from build123d import *

# Parameters (mm, degrees)
BOSS_EXTRUDE1_DEPTH             = 9
SKETCH2_R                       = 15
MOTOR_HOLE_DEPTH                = 123.513264588
CBORE_START                     = -1
CBORE_SLOT_FOR_M3_SHCS1_DEPTH   = 10
CBORE_START_2                   = 6
CBORE_SLOT_FOR_M3_SHCS1_2_DEPTH = 3
LPATTERN2_COUNT                 = 2
LPATTERN2_PITCH                 = 31
LPATTERN2_COUNT_DIR2            = 2
LPATTERN2_PITCH_DIR2            = 31
CBORE_SLOT_FOR_M5_SHCS1_DEPTH   = 5
CBORE_START_3                   = 5
CBORE_SLOT_FOR_M5_SHCS1_2_DEPTH = 4
M5X0_8_TAPPED_HOLE1_D           = 4.2


with BuildPart() as part:
    # Sketch1 → Boss-Extrude1 (new body)
    with BuildSketch(Plane.XY):
        Polygon((-33.5, 0), (33.5, 0), (33.5, 117.5), (-28.5, 117.5), (-33.5, 112.5), align=None)
    extrude(amount=BOSS_EXTRUDE1_DEPTH)

    # Sketch2 → Motor Hole (cut, through all)
    with BuildSketch(Plane.XY.offset(9)):
        with Locations((0, 44.5)):
            Circle(SKETCH2_R)
    extrude(amount=-MOTOR_HOLE_DEPTH, mode=Mode.SUBTRACT)

    # CBORE SLOT for M3 SHCS1: read off the stored shape, not the designer's step
    # CBORE SLOT for M3 SHCS1 outline → CBORE SLOT for M3 SHCS1 (cut)
    with BuildSketch(Plane.XY.offset(CBORE_START)):
        with BuildLine():
            Line((-13.8, 55.2), (-13.8, 65.3))
            ThreePointArc((-13.8, 65.3), (-15.5, 67), (-17.2, 65.3))
            Line((-17.2, 65.3), (-17.2, 55.2))
            ThreePointArc((-17.2, 55.2), (-15.5, 53.5), (-13.8, 55.2))
        make_face()
    cbore_slot_for_m3_shcs1 = extrude(amount=CBORE_SLOT_FOR_M3_SHCS1_DEPTH, mode=Mode.SUBTRACT)

    # CBORE SLOT for M3 SHCS1 2 outline → CBORE SLOT for M3 SHCS1 2 (cut)
    with BuildSketch(Plane.XY.offset(CBORE_START_2)):
        with BuildLine():
            Line((-12.25, 55.2), (-12.25, 65.3))
            ThreePointArc((-12.25, 65.3), (-15.5, 68.55), (-18.75, 65.3))
            Line((-18.75, 65.3), (-18.75, 55.2))
            ThreePointArc((-18.75, 55.2), (-15.5, 51.95), (-12.25, 55.2))
        make_face()
        with BuildLine():
            ThreePointArc((-17.2, 65.3), (-15.5, 67), (-13.8, 65.3))
            Line((-13.8, 65.3), (-13.8, 55.2))
            ThreePointArc((-13.8, 55.2), (-15.5, 53.5), (-17.2, 55.2))
            Line((-17.2, 55.2), (-17.2, 65.3))
        make_face(mode=Mode.SUBTRACT)
    cbore_slot_for_m3_shcs1_2 = extrude(amount=CBORE_SLOT_FOR_M3_SHCS1_2_DEPTH, mode=Mode.SUBTRACT)

    # CBORE SLOT for M3 SHCS1 3: loft between two sections, ruled curve by curve
    cbore_slot_for_m3_shcs1_3_from = [
        Edge.make_three_point_arc((-12.25, 65.3, 8.975), (-13.201902961, 67.598097039, 8.975), (-15.5, 68.55, 8.975)),
        Edge.make_three_point_arc((-15.5, 68.55, 8.975), (-17.798097039, 67.598097039, 8.975), (-18.75, 65.3, 8.975)),
        Edge.make_three_point_arc((-18.75, 55.2, 8.975), (-17.798097039, 52.901902961, 8.975), (-15.5, 51.95, 8.975)),
        Edge.make_three_point_arc((-15.5, 51.95, 8.975), (-13.201902961, 52.901902961, 8.975), (-12.25, 55.2, 8.975)),
        Edge.make_line((-18.75, 65.3, 8.975), (-18.75, 55.2, 8.975)),
        Edge.make_line((-12.25, 65.3, 8.975), (-12.25, 55.2, 8.975)),
    ]
    cbore_slot_for_m3_shcs1_3_to = [
        Edge.make_three_point_arc((-12.225, 65.3, 9), (-13.184225292, 67.615774708, 9), (-15.5, 68.575, 9)),
        Edge.make_three_point_arc((-15.5, 68.575, 9), (-17.815774708, 67.615774708, 9), (-18.775, 65.3, 9)),
        Edge.make_three_point_arc((-18.775, 55.2, 9), (-17.815774708, 52.884225292, 9), (-15.5, 51.925, 9)),
        Edge.make_three_point_arc((-15.5, 51.925, 9), (-13.184225292, 52.884225292, 9), (-12.225, 55.2, 9)),
        Edge.make_line((-18.775, 65.3, 9), (-18.775, 55.2, 9)),
        Edge.make_line((-12.225, 65.3, 9), (-12.225, 55.2, 9)),
    ]
    cbore_slot_for_m3_shcs1_3 = Solid(Shell([*[Face.make_surface_from_curves(cbore_slot_for_m3_shcs1_3_from[k], cbore_slot_for_m3_shcs1_3_to[k]) for k in range(6)], Face(Wire(cbore_slot_for_m3_shcs1_3_from)), Face(Wire(cbore_slot_for_m3_shcs1_3_to))]))
    add(cbore_slot_for_m3_shcs1_3, mode=Mode.SUBTRACT)

    # LPattern2: CBORE SLOT for M3 SHCS1, CBORE SLOT for M3 SHCS1 2, CBORE SLOT for M3 SHCS1 3 2 × 2
    with Locations(*[(i * LPATTERN2_PITCH, -j * LPATTERN2_PITCH_DIR2, 0) for i in range(LPATTERN2_COUNT) for j in range(LPATTERN2_COUNT_DIR2) if (i, j) != (0, 0)]):
        add(cbore_slot_for_m3_shcs1, mode=Mode.SUBTRACT)
        add(cbore_slot_for_m3_shcs1_2, mode=Mode.SUBTRACT)
        add(cbore_slot_for_m3_shcs1_3, mode=Mode.SUBTRACT)

    # CBORE SLOT for M5 SHCS1: read off the stored shape, not the designer's step
    # CBORE SLOT for M5 SHCS1 outline → CBORE SLOT for M5 SHCS1 (cut)
    with BuildSketch(Plane.XY):
        with BuildLine():
            ThreePointArc((20.5, 42.5), (25.5, 37.5), (30.5, 42.5))
            Line((30.5, 42.5), (30.5, 57.5))
            ThreePointArc((30.5, 57.5), (25.5, 62.5), (20.5, 57.5))
            Line((20.5, 57.5), (20.5, 42.5))
        make_face()
    cbore_slot_for_m5_shcs1 = extrude(amount=CBORE_SLOT_FOR_M5_SHCS1_DEPTH, mode=Mode.SUBTRACT)

    # CBORE SLOT for M5 SHCS1 2 outline → CBORE SLOT for M5 SHCS1 2 (cut)
    with BuildSketch(Plane.XY.offset(CBORE_START_3)):
        with BuildLine():
            ThreePointArc((22.75, 42.5), (25.5, 39.75), (28.25, 42.5))
            Line((28.25, 42.5), (28.25, 57.5))
            ThreePointArc((28.25, 57.5), (25.5, 60.25), (22.75, 57.5))
            Line((22.75, 57.5), (22.75, 42.5))
        make_face()
    cbore_slot_for_m5_shcs1_2 = extrude(amount=CBORE_SLOT_FOR_M5_SHCS1_2_DEPTH, mode=Mode.SUBTRACT)

    # CBORE SLOT for M5 SHCS1 3: loft between two sections, ruled curve by curve
    cbore_slot_for_m5_shcs1_3_from = [
        Edge.make_three_point_arc((30.5, 42.5, 0.025), (29.035533906, 38.964466094, 0.025), (25.5, 37.5, 0.025)),
        Edge.make_three_point_arc((25.5, 37.5, 0.025), (21.964466094, 38.964466094, 0.025), (20.5, 42.5, 0.025)),
        Edge.make_three_point_arc((20.5, 57.5, 0.025), (21.964466094, 61.035533906, 0.025), (25.5, 62.5, 0.025)),
        Edge.make_three_point_arc((25.5, 62.5, 0.025), (29.035533906, 61.035533906, 0.025), (30.5, 57.5, 0.025)),
        Edge.make_line((20.5, 42.5, 0.025), (20.5, 57.5, 0.025)),
        Edge.make_line((30.5, 42.5, 0.025), (30.5, 57.5, 0.025)),
    ]
    cbore_slot_for_m5_shcs1_3_to = [
        Edge.make_three_point_arc((30.525, 42.5, 0), (29.053211575, 38.946788425, 0), (25.5, 37.475, 0)),
        Edge.make_three_point_arc((25.5, 37.475, 0), (21.946788425, 38.946788425, 0), (20.475, 42.5, 0)),
        Edge.make_three_point_arc((20.475, 57.5, 0), (21.946788425, 61.053211575, 0), (25.5, 62.525, 0)),
        Edge.make_three_point_arc((25.5, 62.525, 0), (29.053211575, 61.053211575, 0), (30.525, 57.5, 0)),
        Edge.make_line((20.475, 42.5, 0), (20.475, 57.5, 0)),
        Edge.make_line((30.525, 42.5, 0), (30.525, 57.5, 0)),
    ]
    cbore_slot_for_m5_shcs1_3 = Solid(Shell([*[Face.make_surface_from_curves(cbore_slot_for_m5_shcs1_3_from[k], cbore_slot_for_m5_shcs1_3_to[k]) for k in range(6)], Face(Wire(cbore_slot_for_m5_shcs1_3_from)), Face(Wire(cbore_slot_for_m5_shcs1_3_to))]))
    add(cbore_slot_for_m5_shcs1_3, mode=Mode.SUBTRACT)

    # Mirror1: CBORE SLOT for M5 SHCS1, CBORE SLOT for M5 SHCS1 2, CBORE SLOT for M5 SHCS1 3 across plane
    add(cbore_slot_for_m5_shcs1.mirror(Plane(origin=(0, 0, 0), x_dir=(0, 0, 1), z_dir=(1, 0, 0))), mode=Mode.SUBTRACT)
    add(cbore_slot_for_m5_shcs1_2.mirror(Plane(origin=(0, 0, 0), x_dir=(0, 0, 1), z_dir=(1, 0, 0))), mode=Mode.SUBTRACT)
    add(cbore_slot_for_m5_shcs1_3.mirror(Plane(origin=(0, 0, 0), x_dir=(0, 0, 1), z_dir=(1, 0, 0))), mode=Mode.SUBTRACT)

    # M5x0.8 Tapped Hole1 (through all)
    with Locations(Plane.XY.offset(9)):
        with Locations((23.5, 94), (23.5, 80)):
            Hole(M5X0_8_TAPPED_HOLE1_D / 2)


solid = part.part
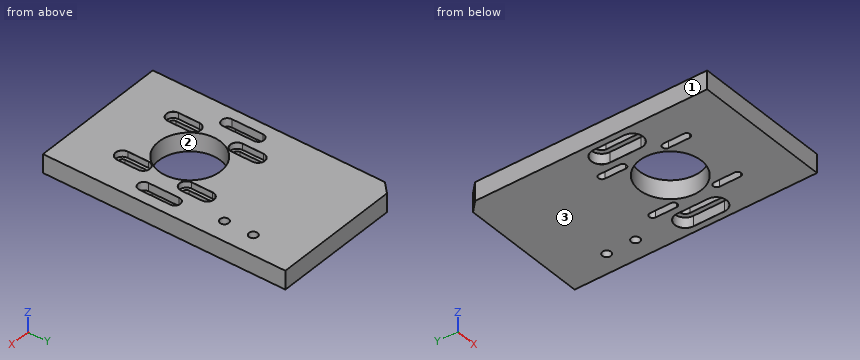
CAD build for the part. Positions are in the model's coordinates, mm. Face numbers are marked on the shaded views. Round coordinates to 2 decimals unless told otherwise and drop trailing zeros. Write each loop counter-clockwise with the first axis right and the second up, starting at its lowest first coordinate (ties: lowest second). Pieces come first, ordered by that corner, then holes.
(1) Slice it at B-B, the plane z = 3. Count the separate pieces of the cut face and the enclosed holes in it, and give its area (3 significant figures).
(2) Probe line 1 along Y through (x, z) = (0, 2.75); line 2 along Y through (x, z) = (23.5, 3.5); line 3 along X through (y, z) = (60, 5.25). List the from-to ranges inside material, lowest first.
(3) Slice it at A-A, the plane y = 94. Write the cut outline in (x, z), and give its area (3 significant figures).
(4) Slice it at C-C, the plane x = 10.5. Write the cut outline in (y, z), and give its area (3 significant figures).
(5) Drop flat-ended pins along their axis: P1, Ø5, axis at x = -27.5, y = 47, coming from the -Z side; P2, Ø2, axis at x = -16, y = 63.5, coming from the +Z side. Give the stop position or say it passes through.
(6) Mould opens along X. For the marked faces 1, 2 and 3 say: pulls with the +X half, pulls with the -X half, needs draft (parallel to the pull), parting line crosses it, or undercut.
From the geometry:
1. separate pieces: 1
1. enclosed holes: 9
1. area: 6,490 mm2
2. line 1: y = 0 to 29.5, 59.5 to 117.5
2. line 2: y = 0 to 37.92, 62.08 to 77.9, 82.1 to 91.9, 96.1 to 117.5
2. line 3: x = -33.5 to -26.65, -24.35 to -17.2, -13.8 to 13.8, 17.2 to 24.35, 26.65 to 33.5
3. outline: (-33.5, 0) - (21.4, 0) - (21.4, 9) - (-33.5, 9) - close; (25.6, 0) - (33.5, 0) - (33.5, 9) - (25.6, 9) - close
3. area: 565 mm2
4. outline: (0, 0) - (33.79, 0) - (33.79, 9) - (0, 9) - close; (55.21, 0) - (117.5, 0) - (117.5, 9) - (55.21, 9) - close
4. area: 865 mm2
5. P1: stops at z = 5
5. P2: passes through
6. face 1: pulls with the -X half
6. face 2: undercut
6. face 3: needs draft
